Part model, mm, in its own coordinate system. Give positions to 0.01 mm unless a question says otherwise; leave off trailing zeros. Write each loop counter-clockwise with the first axis right and the second up, starting at its lowest first coordinate (ties: lowest second). Pieces come first, ordered by that corner, then holes. Notation, with made-up numbers: (60, 4) - (71, 4) arc R22 ccw to (71, 42) - close; hole circle Ø6 at (49, 56). An arc over 180 degrees is marked (long way). Answer in a Markdown table with one row per item. Add a question column.
1. Probe line 1 along Z through (x, y) = (-21, -944); line 2 along X through (y, z) = (-1327, 1.25); line 3 along Z through (x, y) = (0.5, -670). List the from-to ranges inside material, lowest first.
2. Drop flat-ended pins along their axis: pin 1 Ø4 at (x, y) = (-23, -724) entering from +Z; pin 2 Ø2 at (x, y) = (-17, -690.5) entering from +Z; pin 3 Ø0.5 at (y, z) = (-1104.5, 0.5) entering from -X. Give the stop position or say it passes through.
3. Band-saw the part on B-B on x = -9. Write the cut outline in (y, z) (1 decimal), plus the area to 3 significant figures.
```python
from build123d import *

# Parameters (mm, degrees)
F1_DEPTH = 1546.225
F2_R     = 76.2
F3_R     = 3.175
F4_R     = 3.175


with BuildPart() as f1:
    # F0 (on Front) → F1 (new body)
    with BuildSketch(Plane.XZ):
        Polygon((-10.945544, 11.1125), (-31.677012, 5.55752), (-31.677012, 1.5875), (3.247988, 1.5875), (3.247988, 0), (19.122988, 0), (19.122988, 11.1125), align=None)
    extrude(amount=F1_DEPTH)

    # F2
    f2_edges = [f1.edges().sort_by_distance(p)[0] for p in [
        (-10.945544, -773.1125, 11.1125),
    ]]
    fillet(f2_edges, radius=F2_R)

    # F3
    f3_edges = [f1.edges().sort_by_distance(p)[0] for p in [
        (-31.677012, -773.1125, 5.55752),
    ]]
    fillet(f3_edges, radius=F3_R)

    # F4
    f4_edges = [f1.edges().sort_by_distance(p)[0] for p in [
        (19.122988, -773.1125, 11.1125),
    ]]
    fillet(f4_edges, radius=F4_R)


solid = f1.part
```
Values:
| question | item | result |
|---|---|---|
| 1 | line 1 | z = 1.59 to 8.42 |
| 1 | line 2 | x = 3.25 to 19.12 |
| 1 | line 3 | z = 1.59 to 11.11 |
| 2 | pin 1 | stops at z = 8.42 |
| 2 | pin 2 | stops at z = 9.6 |
| 2 | pin 3 | stops at x = 3.25 |
| 3 | outline | (-1546.2, 1.6) - (0, 1.6) - (0, 10.7) - (-1546.2, 10.7) - close |
| 3 | area | 14,100 mm² |
